Geometry check sheet. Reference: the model listing, model coordinates, mm. Give positions to 0.01 mm unless a question says otherwise; leave off trailing zeros. Loops run counter-clockwise (first coordinate to the right, second up) from the corner with the lowest first, then second, coordinate; pieces in that order, holes last. Notation, with made-up numbers: (83, -23) -> (120, -23) arc R23 ccw to (120, 6) -> close; hole circle Ø3 at (14.5, 39). An arc over 180 degrees is marked (long way). Answer as a JSON object with one key per item and string values.
from build123d import *

# Parameters (mm, degrees)
SKETCH1_R           = 57.5
SKETCH1_R_2         = 15.125
SKETCH1_R_3         = 2.25
BOSS_EXTRUDE1_DEPTH = 5
SKETCH3_R           = 1.7
CUT_EXTRUDE1_DEPTH  = 82.470853684


with BuildPart() as part:
    # Sketch1 → Boss-Extrude1 (new body)
    with BuildSketch(Plane(origin=(0, 0, 0), x_dir=(1, 0, 0), z_dir=(0, 1, 0))):
        with Locations(Location((0, 0, 0), (0, 0, 270))):
            Circle(SKETCH1_R)
        with Locations(Location((0, 0, 0), (0, 0, 270))):
            Circle(SKETCH1_R_2, mode=Mode.SUBTRACT)
        with Locations(Location((5.699343677, -28.434441821, 0), (0, 0, 270))):
            Circle(SKETCH1_R_3, mode=Mode.SUBTRACT)
        with Locations(Location((33.29135337, -22.173989059, 0), (0, 0, 270))):
            Circle(SKETCH1_R_3, mode=Mode.SUBTRACT)
        with Locations(Location((-28.434441821, -5.699343677, 0), (0, 0, 270))):
            Circle(SKETCH1_R_3, mode=Mode.SUBTRACT)
        with Locations(Location((-22.173989059, -33.29135337, 0), (0, 0, 270))):
            Circle(SKETCH1_R_3, mode=Mode.SUBTRACT)
        with Locations(Location((-5.699343677, 28.434441821, 0), (0, 0, 270))):
            Circle(SKETCH1_R_3, mode=Mode.SUBTRACT)
        with Locations(Location((-33.29135337, 22.173989059, 0), (0, 0, 270))):
            Circle(SKETCH1_R_3, mode=Mode.SUBTRACT)
        with Locations(Location((28.434441821, 5.699343677, 0), (0, 0, 270))):
            Circle(SKETCH1_R_3, mode=Mode.SUBTRACT)
        with Locations(Location((22.173989059, 33.29135337, 0), (0, 0, 270))):
            Circle(SKETCH1_R_3, mode=Mode.SUBTRACT)
    extrude(amount=BOSS_EXTRUDE1_DEPTH)

    # Sketch3 → Cut-Extrude1 (cut, through all)
    with BuildSketch(Plane(origin=(0, 5, 0), x_dir=(1, 0, 0), z_dir=(0, 1, 0))):
        with Locations(Location((0, 24, 0), (0, 0, 270))):
            Circle(SKETCH3_R)
        with Locations(Location((20.784609691, -12, 0), (0, 0, 270))):
            Circle(SKETCH3_R)
        with Locations(Location((-20.784609691, -12, 0), (0, 0, 270))):
            Circle(SKETCH3_R)
    extrude(amount=-CUT_EXTRUDE1_DEPTH, mode=Mode.SUBTRACT)


solid = part.part
1) Section check B-B on z = 0. Record the cut outline in (x, y) (3 decimals), plus the area to 3 significant figures.
Geometry check:
{"outline": "(-57.5, 0) -> (-15.125, 0) -> (-15.125, 5) -> (-57.5, 5) -> close; (15.125, 0) -> (57.5, 0) -> (57.5, 5) -> (15.125, 5) -> close", "area": "424 mm2"}
2) Section check A-A on x = 0. Record the cut outline in (y, z) (3 decimals), plus the area to 3 significant figures.
Geometry check:
{"outline": "(0, -57.5) -> (5, -57.5) -> (5, -25.7) -> (0, -25.7) -> close; (0, -22.3) -> (5, -22.3) -> (5, -15.125) -> (0, -15.125) -> close; (0, 15.125) -> (5, 15.125) -> (5, 57.5) -> (0, 57.5) -> close", "area": "407 mm2"}
3) Section check D-D on z = 12. Record the cut outline in (x, y), plus the area to 3 significant figures.
Geometry check:
{"outline": "(-56.23, 0) -> (-22.48, 0) -> (-22.48, 5) -> (-56.23, 5) -> close; (-19.08, 0) -> (-9.21, 0) -> (-9.21, 5) -> (-19.08, 5) -> close; (9.21, 0) -> (19.08, 0) -> (19.08, 5) -> (9.21, 5) -> close; (22.48, 0) -> (56.23, 0) -> (56.23, 5) -> (22.48, 5) -> close", "area": "436 mm2"}
4) Draft check along Z on faces 1 (the face through (-26.914, 2.465, 4.041)), 2 (the face through (-56.133, 2.465, -12.465)), 3 (the face through (31.92, 2.46, 20.39)), 4 (the face through (-12, 0, 12)). Enter one of: pulls with the +Z half, pulls with the -Z half, needs draft (parallel to the pull), parting line crosses it, or undercut.
Geometry check:
{"face 1": "undercut", "face 2": "parting line crosses it", "face 3": "undercut", "face 4": "needs draft"}
5) Material ranges on line 1 along Z through (x, y) = (4, 4.3); line 2 along X through (y, z) = (1.4, 7.5); line 3 along Z through (x, y) = (-21, 1.4), recorded low to high. Write a range as from..to.
Geometry check:
{"line 1": "z = -57.36..-14.59, 14.59..26.96, 29.91..57.36", "line 2": "x = -57.01..-29.78, -27.09..-13.13, 13.13..57.01", "line 3": "z = -53.53..10.31, 13.69..31.37, 35.21..53.53"}
6) Section check C-C on y = 1.2. Count the separate pieces of the cut face and the enclosed holes in it, plus the area to 3 significant figures.
Geometry check:
{"separate pieces": "1", "enclosed holes": "12", "area": "9,510 mm2"}
7) Depth check by flat-ended pin: P1, Ø5, axis at x = -28.43, z = 5.7, coming from the -Y side; P2, Ø2.5, axis at x = -20.78, z = 12, coming from the -Y side; P3, Ø1, axis at x = 33, y = 2.5, coming from the -Z side; P4, Ø1.5, axis at y = 1.5, z = 13, coming from the +X side. Enter the tip coordinate at first touch or a pass-through.
Geometry check:
{"P1": "stops at y = 0", "P2": "passes through", "P3": "stops at z = -47.43", "P4": "stops at x = 56.18"}
